Input: part model. Units: mm. Frame: model coordinates. Face numbers are marked on the shaded views. Coordinates: 2 decimals unless noted, no trailing zeros. Write each loop counter-clockwise with the first axis right and the second up, starting at its lowest first coordinate (ties: lowest second). Pieces come first, ordered by that corner, then holes. Notation, with made-up numbers: M -1,15.25 L 3,15.25 A25 cw 3,35.25 Z; hole C 84.25,47 d5. An arc over 180 degrees is marked long. Answer as a JSON object with one key per item and string values. Group by question number.
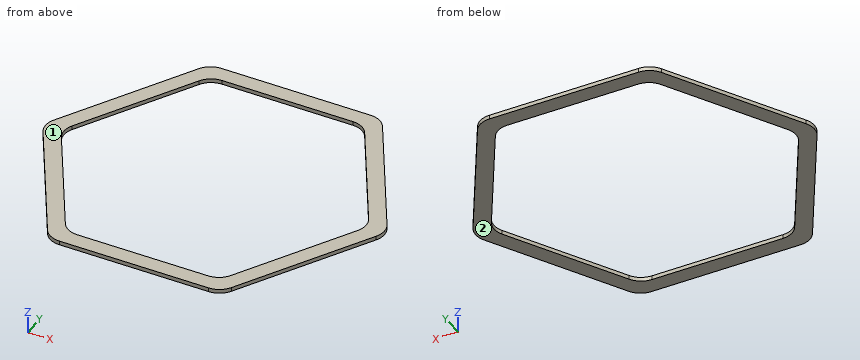
Autodesk Inventor part; units mm, degrees
ref_plane "YZ Plane" through (0, 0, 0) normal (1, 0, 0) x (0, 1, 0)
ref_plane "XZ Plane" through (0, 0, 0) normal (0, 1, 0) x (-1, 0, 0)
ref_plane "XY Plane" through (0, 0, 0) normal (0, 0, 1) x (1, 0, 0)
sketch "Sketch1" plane through (0, 0, 0) normal (0, 0, 1) x (1, 0, 0)
  line L0 (43.3013, -75) -> (-43.3013, -75)
  line L1 (-43.3013, -75) -> (-86.6025, 0)
  line L2 (-86.6025, 0) -> (-43.3013, 75)
  line L3 (-43.3013, 75) -> (43.3013, 75)
  line L4 (43.3013, 75) -> (86.6025, 0)
  line L5 (86.6025, 0) -> (43.3013, -75)
  point P0 (0, 0)
  point P1 (0, 0)
  dimension "d0" = 150
extrude "Extrusion1" add sketch "Sketch1" along normal blind 2
sketch "Sketch7" plane through (0, 0, 2) normal (0, 0, 1) x (1, 0, 0)
  line L0 (40.9919, 71) -> (-40.9919, 71)
  line L1 (-40.9919, 71) -> (-81.9837, 0)
  line L2 (-81.9837, 0) -> (-40.9919, -71)
  line L3 (-40.9919, -71) -> (40.9919, -71)
  line L4 (40.9919, -71) -> (81.9837, 0)
  line L5 (81.9837, 0) -> (40.9919, 71)
  line L6 (-38.6825, -67) -> (-77.3649, 0)
  line L7 (-77.3649, 0) -> (-38.6825, 67)
  line L8 (-38.6825, 67) -> (38.6825, 67)
  line L9 (38.6825, 67) -> (77.3649, 0)
  line L10 (77.3649, 0) -> (38.6825, -67)
  line L11 (38.6825, -67) -> (-38.6825, -67)
  point P0 (0, 0)
  dimension "d19" = 4
extrude "Extrusion6" cut sketch "Sketch7" against normal blind 7 contours L6 L7 L8 L9 L10 L11
fillet "Fillet2" radius 10 6 edges at (38.6825, -67, 1) (77.3649, 0, 1) (38.6825, 67, 1) (-38.6825, 67, 1) (-77.3649, 0, 1) (-38.6825, -67, 1)
fillet "Fillet3" radius 10 6 edges at (-43.3013, 75, 1) (43.3013, 75, 1) (86.6025, 0, 1) (43.3013, -75, 1) (-43.3013, -75, 1) (-86.6025, 0, 1)
properties part number "Cover v1"
Q1. Section C-C, the plane y = -43. Return the cut outline in (x, z).
Q2. Section A-A, the plane x = 17. Return the cut outline in (y, z).
Q3. Section B-B, the plane z = 1.7. Return the cut outline in (x, y), and give its area (3 significant figures).
Q4. Line query: line 1 (Y direction, x = 31.5, z = 0.85); line 2 (X direction, y = -1, z = 1.6); line 3 (X direction, y = -3, z = 1.7). Output: solid intervals per line, ascending. Write a range as from..to.
Q5. Draft query along Z for the marked faces 1 and 2. Return one class per face: released by +Z, released by -Z, zero draft, split by the parting line, or undercut.
Filled in:
{
 "1": {"outline": "M -61.78,0 L -52.54,0 L -52.54,2 L -61.78,2 Z; M 52.54,0 L 61.78,0 L 61.78,2 L 52.54,2 Z"},
 "2": {"outline": "M -75,0 L -67,0 L -67,2 L -75,2 Z; M 67,0 L 75,0 L 75,2 L 67,2 Z"},
 "3": {"outline": "M -83.72,-5 L -46.19,-70 A10 ccw -37.53,-75 L 37.53,-75 A10 ccw 46.19,-70 L 83.72,-5 A10 ccw 83.72,5 L 46.19,70 A10 ccw 37.53,75 L -37.53,75 A10 ccw -46.19,70 L -83.72,5 A10 ccw Z; hole M -74.48,-5 L -41.57,-62 A10 ccw -32.91,-67 L 32.91,-67 A10 ccw 41.57,-62 L 74.48,-5 A10 ccw 74.48,5 L 41.57,62 A10 ccw 32.91,67 L -32.91,67 A10 ccw -41.57,62 L -74.48,5 A10 ccw Z", "area": "3,940 mm^2"},
 "4": {"line 1": "-75..-67, 67..75", "line 2": "-85.01..-75.77, 75.77..85.01", "line 3": "-84.59..-75.36, 75.36..84.59"},
 "5": {"face 1": "released by +Z", "face 2": "released by -Z"}
}
